Geometry check sheet. Reference: the model listing, model coordinates, mm. Face numbers are marked on the shaded views. A direction names the side the tool comes from. Round coordinates to 2 decimals unless told otherwise and drop trailing zeros. Order: outer loops, then holes, each group sorted by start corner. A loop starts at its lowest first (then second) coordinate and runs counter-clockwise, first axis right, second up. Notation, with made-up numbers: (-27, 39) - (31, 39) arc R22 cw to (31, 60) - close; hole circle Ø8 at (49.5, 70.25). An arc over 180 degrees is marked (long way). Write each question's results on one line, items separated by ' | '.
```python
from build123d import *

# Parameters (mm, degrees)
SKETCH_W             = 110
SKETCH_H             = 70
PAD_DEPTH            = 3
SKETCH001_W          = 2
SKETCH001_H          = 52
PAD001_DEPTH         = 35
SKETCH002_W          = 10
SKETCH002_H          = 45
PAD002_DEPTH         = 52
SKETCH003_W          = 110
SKETCH003_H          = 5
PAD003_DEPTH         = 52
SKETCH004_R          = 3.5
SKETCH004_W          = 43.5
SKETCH004_H          = 37
POCKET_DEPTH         = 5
SKETCH005_R          = 2.5
POCKET001_DEPTH      = 10
SKETCH006_R          = 6
POCKET002_DEPTH      = 5
SKETCH011_R          = 6
POCKET003_DEPTH      = 150
SKETCH007_R          = 1.65
POCKET004_DEPTH      = 5
POCKET005_DEPTH      = 1.4
SKETCH009_W          = 3.3
SKETCH009_H          = 5.715768
POCKET006_DEPTH      = 0.2
SKETCH010_W          = 3.3
SKETCH010_H          = 3.3
POCKET007_DEPTH      = 0.2
CHAMFER_SIZE         = 5
POCKET012_DEPTH      = 5
BODY_PLACEMENT_ANGLE = 90


with BuildPart() as part:
    # Sketch → Pad (new body)
    with BuildSketch(Plane.XZ):
        Rectangle(SKETCH_W, SKETCH_H)
    extrude(amount=PAD_DEPTH)

    # Sketch001 → Pad001 (join, symmetric)
    with BuildSketch(Plane.XY):
        with Locations((54, -26)):
            Rectangle(SKETCH001_W, SKETCH001_H)
        with Locations((-54, -26)):
            Rectangle(SKETCH001_W, SKETCH001_H)
    extrude(amount=PAD001_DEPTH, both=True)

    # Sketch002 → Pad002 (join)
    with BuildSketch(Plane.XZ):
        with Locations((50, 12.5)):
            Rectangle(SKETCH002_W, SKETCH002_H)
    extrude(amount=PAD002_DEPTH)

    # Sketch003 → Pad003 (join)
    with BuildSketch(Plane.XZ):
        with Locations((0, -7.5)):
            Rectangle(SKETCH003_W, SKETCH003_H)
    extrude(amount=PAD003_DEPTH)

    # Sketch004 (on Face19 of Pad003) → Pocket (cut)
    with BuildSketch(Plane(origin=(0, 0, -5), x_dir=(-1, 0, 0), z_dir=(0, 0, 1))):
        with Locations((29.25, 34.5)):
            Circle(SKETCH004_R)
        with Locations((-15.25, 33.5)):
            Rectangle(SKETCH004_W, SKETCH004_H)
    extrude(amount=-POCKET_DEPTH, mode=Mode.SUBTRACT)

    # Sketch005 (on Face20 of Pocket) → Pocket001 (cut)
    with BuildSketch(Plane(origin=(45, 0, 0), x_dir=(0, 0, -1), z_dir=(-1, 0, 0))):
        with Locations((-19, 27.5)):
            Circle(SKETCH005_R)
    extrude(amount=-POCKET001_DEPTH, mode=Mode.SUBTRACT)

    # Sketch006 (on Face20 of Pocket001) → Pocket002 (cut)
    with BuildSketch(Plane(origin=(45, 0, 0), x_dir=(0, 0, -1), z_dir=(-1, 0, 0))):
        with Locations((-19, 27.5)):
            Circle(SKETCH006_R)
    extrude(amount=-POCKET002_DEPTH, mode=Mode.SUBTRACT)

    # Sketch011 (on Face20 of Pocket002) → Pocket003 (cut)
    with BuildSketch(Plane(origin=(45, 0, 0), x_dir=(0, 0, -1), z_dir=(-1, 0, 0))):
        with Locations((-19, 27.5)):
            Circle(SKETCH011_R)
    extrude(amount=POCKET003_DEPTH, mode=Mode.SUBTRACT)

    # Sketch007 → Pocket004 (cut)
    with BuildSketch(Plane.XZ):
        with Locations((-27, -16.5)):
            Circle(SKETCH007_R)
        with Locations((27, -16.5)):
            Circle(SKETCH007_R)
    extrude(amount=POCKET004_DEPTH, mode=Mode.SUBTRACT)

    # Sketch008 → Pocket005 (cut)
    with BuildSketch(Plane.XZ):
        Polygon((-25.35, -13.642116), (-28.65, -13.642116), (-30.3, -16.5), (-28.65, -19.357884), (-25.35, -19.357884), (-23.7, -16.5), align=None)
        Polygon((30.3, -16.5), (28.65, -13.642116), (25.35, -13.642116), (23.7, -16.5), (25.35, -19.357884), (28.65, -19.357884), align=None)
    extrude(amount=POCKET005_DEPTH, mode=Mode.SUBTRACT)

    # Sketch009 (on Face67 of Pocket005) → Pocket006 (cut)
    with BuildSketch(Plane(origin=(0, -1.4, 0), x_dir=(1, 0, 0), z_dir=(0, 1, 0))):
        with Locations((-27, 16.5)):
            Rectangle(SKETCH009_W, SKETCH009_H)
        with Locations((27, 16.5)):
            Rectangle(SKETCH009_W, SKETCH009_H)
    extrude(amount=-POCKET006_DEPTH, mode=Mode.SUBTRACT)

    # Sketch010 (on Face95 of Pocket006) → Pocket007 (cut)
    with BuildSketch(Plane(origin=(0, -1.6, 0), x_dir=(1, 0, 0), z_dir=(0, 1, 0))):
        with Locations((27, 16.5)):
            Rectangle(SKETCH010_W, SKETCH010_H)
        with Locations((-27, 16.5)):
            Rectangle(SKETCH010_W, SKETCH010_H)
    extrude(amount=-POCKET007_DEPTH, mode=Mode.SUBTRACT)

    # Chamfer
    chamfer_edges = [part.edges().sort_by_distance(p)[0] for p in [
        (-6.5, -52, -7.5),
        (37, -52, -7.5),
        (-6.5, -15, -7.5),
        (37, -15, -7.5),
    ]]
    chamfer(chamfer_edges, length=CHAMFER_SIZE)

    # Sketch018 → Pocket012 (cut)
    with BuildSketch(Plane.XZ):
        with BuildLine():
            ThreePointArc((-1.5, 9), (-6.5, 4), (-1.5, -1))
            Line((-1.5, -1), (32, -1))
            ThreePointArc((32, -1), (37, 4), (32, 9))
            Line((-1.5, 9), (32, 9))
        make_face()
    extrude(amount=POCKET012_DEPTH, mode=Mode.SUBTRACT)


with BuildPart() as part_1:
    # Body placement: moved
    add(part.part.moved(Location((-112, 118, -67.5))).rotate(Axis((-112, 118, -67.5), (-1, 0, 0)), BODY_PLACEMENT_ANGLE))


solid = part_1.part
```
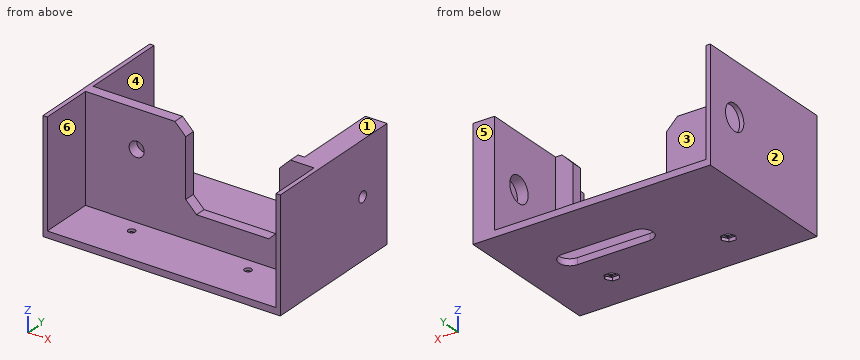
(1) Section check B-B (y = 125). Record the cut outline in (x, z).
Answers follow:
outline: (-167, -67.5) - (-117.5, -67.5) - (-117.5, -64.5) - (-165, -64.5) - (-165, -15.5) - (-167, -15.5) - close; (-76, -67.5) - (-57, -67.5) - (-57, -15.5) - (-67, -15.5) - (-67, -64.5) - (-76, -64.5) - close
(2) Section check D-D (y = 137). Record the cut outline in (x, z), then the cut area to 3 significant figures.
Answers follow:
outline: (-167, -67.5) - (-57, -67.5) - (-57, -42.5) - (-62, -42.5) - (-62, -46) - (-67, -46) - (-67, -64.5) - (-165, -64.5) - (-165, -46) - (-167, -46) - close; (-167, -34) - (-165, -34) - (-165, -15.5) - (-167, -15.5) - close; (-67, -34) - (-62, -34) - (-62, -37.5) - (-57, -37.5) - (-57, -15.5) - (-67, -15.5) - close | area: 809 mm²
(3) Material ranges on line 1 (Y direction, x = -166, z = -40); line 2 (Z direction, x = -166, y = 137); line 3 (X direction, y = 139.5, z = -29.5), recorded low to high.
Answers follow:
line 1: 83 to 131, 143 to 153 | line 2: -67.5 to -46, -34 to -15.5 | line 3: -167 to -165, -67 to -57
(4) Draft check along X on the marked faces 1, 2 and 3. Enter one of: released by +X, released by -X, zero draft, split by the parting line, or undercut.
Answers follow:
face 1: zero draft | face 2: released by -X | face 3: undercut
(5) Section check C-C (x = -101.5). Record the cut outline in (y, z), then the cut area to 3 significant figures.
Answers follow:
outline: (83, -67.5) - (117, -67.5) - (117, -64.5) - (113, -64.5) - (113, -52.5) - (108, -52.5) - (108, -64.5) - (83, -64.5) - close; (127, -67.5) - (153, -67.5) - (153, -64.5) - (127, -64.5) - close | area: 240 mm²
(6) Depth check by flat-ended pin: pin 1 Ø6 at (y, z) = (135.5, -40.5) entering from -X; pin 2 Ø1.8 at (x, y) = (-84, 100.5) entering from -Z; pin 3 Ø5.5 at (x, y) = (-139, 101.5) entering from +Z. Enter the tip coordinate at first touch or a pass-through.
Answers follow:
pin 1: x = -62 | pin 2: z = -66.1 | pin 3: z = -64.5
(7) Section check A-A (z = -27). Record the cut outline in (x, y), then the cut area to 4 significant figures.
Answers follow:
outline: (-167, 83) - (-165, 83) - (-165, 108) - (-118.5, 108) - (-118.5, 113) - (-165, 113) - (-165, 153) - (-167, 153) - close; (-75, 108) - (-59, 108) - (-59, 83) - (-57, 83) - (-57, 153) - (-67, 153) - (-67, 113) - (-75, 113) - close | area: 912.5 mm²
(8) Access from +Z, -Z, +X, -X, +Y, -Y to the whole of each face (thin tool, end or side, straight path). Record for the marked faces 4, 5 and 6.
Answers follow:
face 4: +Z, +Y | face 5: +Z, -Z, +X, -X, +Y | face 6: +Z, -Y
